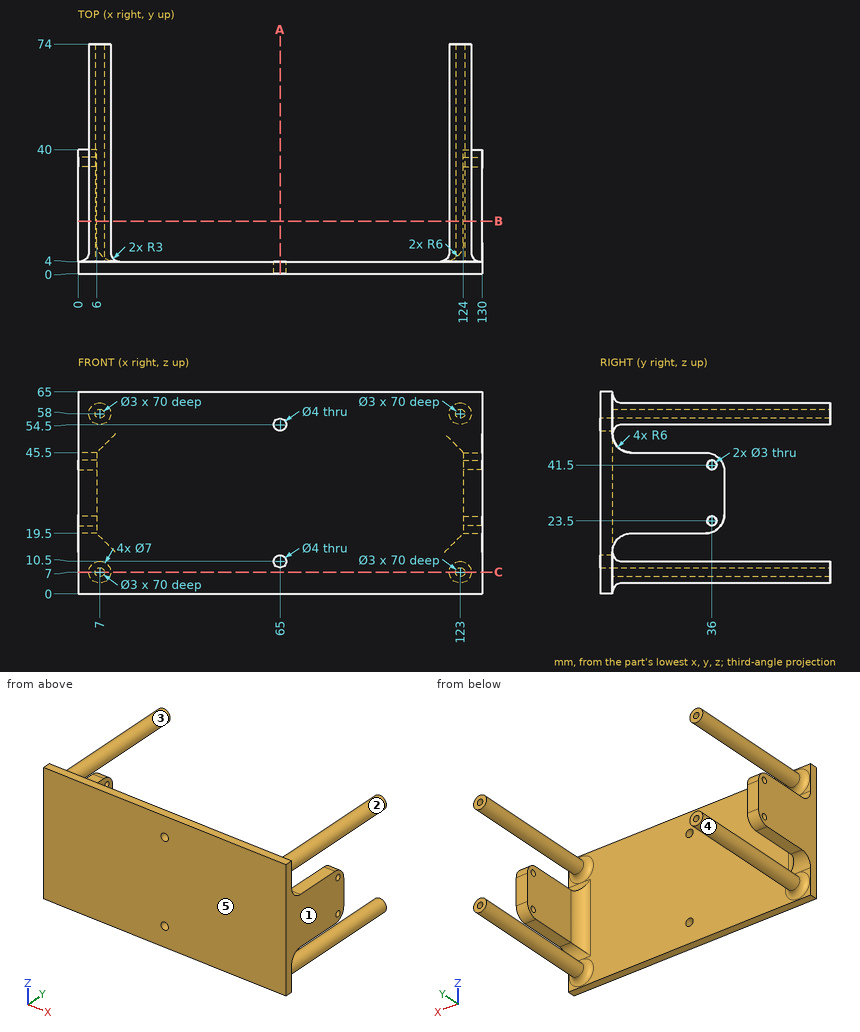
Drawing for the job (mm, zero at the part's lowest x, y, z). A direction names the side the tool comes from. Round coordinates to 2 decimals unless told otherwise and drop trailing zeros. Write each loop counter-clockwise with the first axis right and the second up, starting at its lowest first coordinate (ties: lowest second). Pieces come first, ordered by that corner, then holes.
Item 1: Band-saw the part on C-C on z = 7. Write the cut outline in (x, y).
Filled in:
outline: (0, 0) - (130, 0) - (130, 4) - (129.5, 4) arc R3 cw to (126.5, 7) - (126.5, 74) - (124.5, 74) - (124.5, 4) - (121.5, 4) - (121.5, 74) - (119.5, 74) - (119.5, 7) arc R3 cw to (116.5, 4) - (13.5, 4) arc R3 cw to (10.5, 7) - (10.5, 74) - (8.5, 74) - (8.5, 4) - (5.5, 4) - (5.5, 74) - (3.5, 74) - (3.5, 7) arc R3 cw to (0.5, 4) - (0, 4) - close
Item 2: Band-saw the part on A-A on x = 65. Write the cut outline in (y, z), then the cut area to 3 significant figures.
Filled in:
outline: (0, 0) - (4, 0) - (4, 8.5) - (0, 8.5) - close; (0, 12.5) - (4, 12.5) - (4, 52.5) - (0, 52.5) - close; (0, 56.5) - (4, 56.5) - (4, 65) - (0, 65) - close
area: 228 mm2
Item 3: Band-saw the part on B-B on y = 17. Give the number of separate pieces and of enclosed holes in the cut face, then the cut area to 3 significant figures.
Filled in:
separate pieces: 6
enclosed holes: 4
area: 438 mm2
Item 4: Mould opens along Z. For the marked faces 3, 4 and 5 say: released by +Z, released by -Z, zero draft, split by the parting line, or undercut.
Filled in:
face 3: undercut
face 4: undercut
face 5: zero draft
Item 5: Drill centre lines: L1, parallel to X at y = 53, z = 7; L2, parallel to X at y = 48, z = 6.5; L3, parallel to Y at x = 80, z = 27.5. Where is each one in solid material? Low to high.
Filled in:
L1: x = 3.5 to 5.5, 8.5 to 10.5, 119.5 to 121.5, 124.5 to 126.5
L2: x = 3.54 to 5.59, 8.41 to 10.46, 119.54 to 121.59, 124.41 to 126.46
L3: y = 0 to 4
Item 6: Drop flat-ended pins along their axis: pin 1 Ø1.8 at (x, y) = (2, 27) entering from -Z; pin 2 Ø1.5 at (y, z) = (11, 8.5) entering from -X; pin 3 Ø0.9 at (x, z) = (6.5, 6.5) entering from +Y; pin 4 Ø2.5 at (x, z) = (65, 10.5) entering from -Y. Give the stop position or say it passes through.
Filled in:
pin 1: stops at z = 19.5
pin 2: stops at x = 3.58
pin 3: stops at y = 4
pin 4: passes through
Item 7: Tool access for the marked faces 1 and 2: list every direction of +Z, -Z, +X, -X, +Y, -Y with a clear straight run to the whole face (end or side of a thin tool).
Filled in:
face 1: +Z, -Z, +X, +Y, -Y
face 2: +Y
